For this review, take the finished solid that the model builds, in its own axes (mm). Coordinates: 2 decimals unless noted, no trailing zeros. Loops run counter-clockwise (first coordinate to the right, second up) from the corner with the lowest first, then second, coordinate; pieces in that order, holes last. Notation, with made-up numbers: (49, -22) -> (83, -22) arc R10 cw to (83, -14) -> close; hole circle Ø8 at (47.5, -30). An arc over 180 degrees is marked (long way). Answer in a Markdown table with one row per item.
from build123d import *

# Parameters (mm, degrees)
SKETCH1_R           = 3.25
SKETCH1_R_2         = 0.875
BOSS_EXTRUDE1_DEPTH = 0.25
SKETCH2_R           = 4.078298916
BOSS_EXTRUDE2_DEPTH = 0.25
FILLET1_R           = 1
SHELL1_T            = 0.05
CUT_EXTRUDE1_START  = -2.25
SKETCH3_R           = 0.875
CUT_EXTRUDE1_DEPTH  = 2.25
BOSS_EXTRUDE3_START = 0.25
SKETCH4_R           = 1.213418459
SKETCH4_R_2         = 0.875
BOSS_EXTRUDE3_DEPTH = 0.25
CHAMFER1_SIZE       = 0.2


with BuildPart() as part:
    # Sketch1 → Boss-Extrude1 (new body)
    with BuildSketch(Plane.XY):
        Circle(SKETCH1_R)
        Circle(SKETCH1_R_2, mode=Mode.SUBTRACT)
    extrude(amount=BOSS_EXTRUDE1_DEPTH)

    # Sketch2 → Boss-Extrude2 (add)
    with BuildSketch(Plane(origin=(0, 0, 0), x_dir=(-1, 0, 0), z_dir=(0, 0, -1))):
        Circle(SKETCH2_R)
    extrude(amount=BOSS_EXTRUDE2_DEPTH)

    # Fillet1
    # the kernel refuses this fillet: 1 mm, written as the material it adds along each edge
    with BuildSketch(Plane(origin=(0, 0, 0), x_dir=(1, 0, 0), z_dir=(0, -1, 0))) as fillet1_piece_1:
        with BuildLine():
            CenterArc((3.911437828, 1), FILLET1_R, 228.590377891, 41.409622109)
            Line((3.25, 0.25), (3.25, 0))
            Line((3.25, 0), (3.911437828, 0))
        make_face()
    revolve(axis=Axis((0, 0, 0), (0, 0, 1)))

    # Shell1
    shell1_openings = [part.faces().sort_by_distance(p)[0] for p in [
        (0, 0, -0.25),
    ]]
    offset(amount=SHELL1_T, openings=shell1_openings, kind=Kind.INTERSECTION)

    # Sketch3 → Cut-Extrude1 (cut)
    with BuildSketch(Plane.XY.offset(0.3).offset(CUT_EXTRUDE1_START)):
        Circle(SKETCH3_R)
    extrude(amount=CUT_EXTRUDE1_DEPTH, mode=Mode.SUBTRACT)

    # Sketch4 → Boss-Extrude3 (add)
    with BuildSketch(Plane(origin=(0, 0, 0.25), x_dir=(-1, 0, 0), z_dir=(0, 0, -1)).offset(BOSS_EXTRUDE3_START)):
        with Locations(Location((0, 0, 0), (0, 0, 180))):
            Circle(SKETCH4_R)
        with Locations(Location((0, 0, 0), (0, 0, 180))):
            Circle(SKETCH4_R_2, mode=Mode.SUBTRACT)
    extrude(amount=-BOSS_EXTRUDE3_DEPTH)

    # Chamfer1
    chamfer1_edges = [part.edges().sort_by_distance(p)[0] for p in [
        (-1.213418459, 0, 0),
    ]]
    chamfer(chamfer1_edges, length=CHAMFER1_SIZE)


solid = part.part
Item 1: Insertion check: pin 1 (2.5 mm diameter, centred on x = 0, y = 2, fed in from -Z); pin 2 (1.6 mm diameter, centred on x = 0, y = 0, fed in from -Z); pin 3 (1 mm diameter, centred on x = 2.5, y = -3, fed in from +Z). Each pin has a flat end and moves straight along its axis. Give the tip position at first contact, or say it passes through.
Worked answers:
| item | result |
|---|---|
| pin 1 | z = 0 |
| pin 2 | through |
| pin 3 | z = 0.2 |
Item 2: Take a section at A-A, the plane x = 0. State the section outline as (y, z) points (3 decimals).
Worked answers:
| item | result |
|---|---|
| outline | (-4.128, -0.25) -> (-4.078, -0.25) -> (-4.078, 0) -> (-3.911, 0) arc R1 ccw to (-3.25, 0.25) -> (-1.213, 0.25) -> (-1.213, 0.2) -> (-1.013, 0) -> (-0.875, 0) -> (-0.875, 0.3) -> (-3.269, 0.3) arc R0.95 cw to (-3.911, 0.05) -> (-4.128, 0.05) -> close; (0.875, 0) -> (1.013, 0) -> (1.213, 0.2) -> (1.213, 0.25) -> (3.25, 0.25) arc R1 ccw to (3.911, 0) -> (4.078, 0) -> (4.078, -0.25) -> (4.128, -0.25) -> (4.128, 0.05) -> (3.911, 0.05) arc R0.95 cw to (3.269, 0.3) -> (0.875, 0.3) -> close |
Item 3: For L1, parallel to Z at x = 0.75, y = -0.5, list the stretches that pass through material, from the lowest coordinate up.
Worked answers:
| item | result |
|---|---|
| L1 | 0 to 0.3 |
